Verification items for the finished model (mm, model axes). Face numbers are marked on the shaded views. A direction names the side the tool comes from. Round coordinates to 2 decimals unless told otherwise and drop trailing zeros. Order: outer loops, then holes, each group sorted by start corner. A loop starts at its lowest first (then second) coordinate and runs counter-clockwise, first axis right, second up. Notation, with made-up numbers: M -3.5,23.25 L 55.5,23.25 A35 cw 55.5,57.25 Z; hole C 61.5,73.5 d7. An arc over 180 degrees is marked long. One line per item, written item: value. Start each with the question number.
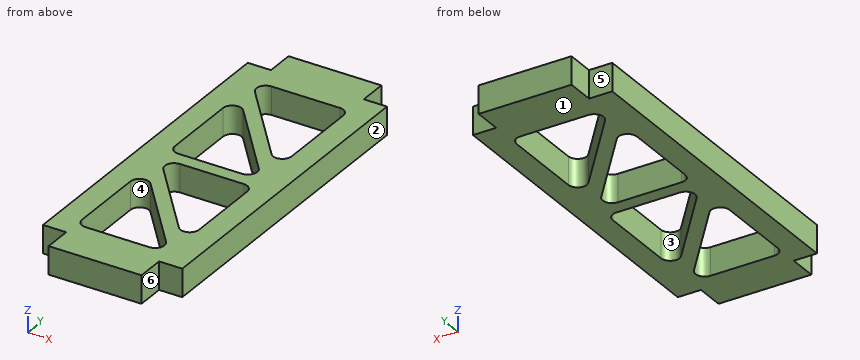
from build123d import *

# Parameters (mm, degrees)
SALIENTE_EXTRUIR1_DEPTH = 3


with BuildPart() as part:
    # Croquis1 → Saliente-Extruir1 (new body)
    with BuildSketch(Plane.XY):
        Polygon((-5, -20.5), (5, -20.5), (5, -17.5), (7.5, -17.5), (7.5, 17.5), (5, 17.5), (5, 20.5), (-5, 20.5), (-5, 17.5), (-7.5, 17.5), (-7.5, -17.5), (-5, -17.5), align=None)
        with BuildLine():
            ThreePointArc((-5, -6.533565594), (-4.340425264, -5.593294017), (-3.23177872, -5.893381195))
            Line((-3.23177872, -5.893381195), (3.638034467, -14.13715702))
            ThreePointArc((3.638034467, -14.13715702), (3.775402609, -15.201496816), (2.869813188, -15.77734142))
            Line((2.869813188, -15.77734142), (-4, -15.77734142))
            ThreePointArc((-4, -15.77734142), (-4.707106781, -15.484448201), (-5, -14.77734142))
            Line((-5, -14.77734142), (-5, -6.533565594))
        make_face(mode=Mode.SUBTRACT)
        with BuildLine():
            ThreePointArc((-3.633179667, -3.068625156), (-3.770547809, -2.00428536), (-2.864958387, -1.428440756))
            Line((-2.864958387, -1.428440756), (4, -1.428440756))
            ThreePointArc((4, -1.428440756), (4.707106781, -1.721333975), (5, -2.428440756))
            Line((5, -2.428440756), (5, -10.666390821))
            ThreePointArc((5, -10.666390821), (4.340425264, -11.606662399), (3.23177872, -11.306575221))
            Line((3.23177872, -11.306575221), (-3.633179667, -3.068625156))
        make_face(mode=Mode.SUBTRACT)
        with BuildLine():
            ThreePointArc((-5, 9.309509308), (-4.340425264, 10.249780886), (-3.23177872, 9.949693708))
            Line((-3.23177872, 9.949693708), (3.633179667, 1.711743643))
            ThreePointArc((3.633179667, 1.711743643), (3.770547809, 0.647403847), (2.864958387, 0.071559244))
            Line((2.864958387, 0.071559244), (-4, 0.071559244))
            ThreePointArc((-4, 0.071559244), (-4.707106781, 0.364452462), (-5, 1.071559244))
            Line((-5, 1.071559244), (-5, 9.309509308))
        make_face(mode=Mode.SUBTRACT)
        with BuildLine():
            Line((3.23177872, 4.536499682), (-4.120984545, 13.3598156))
            ThreePointArc((-4.120984545, 13.3598156), (-4.258352687, 14.424155396), (-3.352763265, 15))
            Line((-3.352763265, 15), (4, 15))
            ThreePointArc((4, 15), (4.707106781, 14.707106781), (5, 14))
            Line((5, 14), (5, 5.176684082))
            ThreePointArc((5, 5.176684082), (4.340425264, 4.236412504), (3.23177872, 4.536499682))
        make_face(mode=Mode.SUBTRACT)
    extrude(amount=SALIENTE_EXTRUIR1_DEPTH)


solid = part.part
1. Scan lines: line 1 along Y through (x, z) = (-3, 0.3); line 2 along Y through (x, z) = (-4.75, 0.4); line 3 along Y through (x, z) = (-4.5, 1.25). Record each from-to range of solid material in increasing order.
2. Depth check by flat-ended pin: pin 1 (1.2 mm diameter, centred on x = -6.5, z = 2, fed in from -Y); pin 2 (0.8 mm diameter, centred on x = 6.5, z = 1.5, fed in from +Y); pin 3 (6 mm diameter, centred on x = -4.5, y = 4, fed in from -Z); pin 4 (1.5 mm diameter, centred on y = -19, z = 1.5, fed in from +X). Enter the tip coordinate at first touch or a pass-through.
3. Draft check along X on the marked faces 1, 2 and 3. Enter one of: released by +X, released by -X, zero draft, split by the parting line, or undercut.
4. Tool access check on the marked faces 4, 5 and 6. Record the directions out of +Z, -Z, +X, -X, +Y, -Y that give a thin tool (end or side, any length) a straight path to the whole face; none if there is none.
5. Section check D-D (y = -5). Record the cut outline in (x, z), and give its area (3 significant figures).
6. Section check A-A (x = 0). Record the cut outline in (y, z).
7. Section check C-C (z = 2.1). Give the number of separate pieces and of enclosed holes in the cut face, and give its area (3 significant figures).
8. Section check B-B (y = 2.5). Record the cut outline in (x, z).
Geometry check:
1. line 1: y = -20.5 to -15.78, -6.17 to -3.83, -1.44 to 0.07, 9.67 to 12.01, 15 to 20.5
1. line 2: y = -20.5 to -15.44, -5.87 to 0.41, 9.97 to 20.5
1. line 3: y = -20.5 to -15.64, -5.67 to 0.21, 10.18 to 20.5
2. pin 1: stops at y = -17.5
2. pin 2: stops at y = 17.5
2. pin 3: stops at z = 0
2. pin 4: stops at x = 5
3. face 1: zero draft
3. face 2: released by +X
3. face 3: undercut
4. face 4: +Z, -Z
4. face 5: +Z, -Z, -X, +Y
4. face 6: +Z, -Z, +X, -Y
5. outline: M -7.5,0 L -2.02,0 L -2.02,3 L -7.5,3 Z; M 5,0 L 7.5,0 L 7.5,3 L 5,3 Z
5. area: 23.9 mm²
6. outline: M -20.5,0 L -15.78,0 L -15.78,3 L -20.5,3 Z; M -9.77,0 L -7.43,0 L -7.43,3 L -9.77,3 Z; M -1.43,0 L 0.07,0 L 0.07,3 L -1.43,3 Z; M 6.07,0 L 8.41,0 L 8.41,3 L 6.07,3 Z; M 15,0 L 20.5,0 L 20.5,3 L 15,3 Z
7. separate pieces: 1
7. enclosed holes: 4
7. area: 350 mm²
8. outline: M -7.5,0 L -5,0 L -5,3 L -7.5,3 Z; M 2.98,0 L 7.5,0 L 7.5,3 L 2.98,3 Z
